Input: part model. Units: mm. Frame: model coordinates. A direction names the side the tool comes from. Coordinates: 2 decimals unless noted, no trailing zeros. Write each loop counter-clockwise with the first axis right and the second up, starting at its lowest first coordinate (ties: lowest second). Pieces come first, ordered by that corner, then holes. Notation, with made-up numbers: M 77.5,38 L 100.5,38 A35 cw 100.5,73 Z; hole C 32,-17 d1. An arc over 180 degrees is marked long. Use CSV: the item, a comma, the result in double quotes.
```python
from build123d import *

# Parameters (mm, degrees)
F0_R     = 5
F0_R_2   = 4.7625
F1_DEPTH = 5
F2_R     = 95
F2_R_2   = 92.5
F3_DEPTH = 38.23
F6_D     = 1.9939
F6_DEPTH = 13.58625
F6_TIP   = 0.5990279941
F7_D     = 10.0838
F7_DEPTH = 13.59
F7_TIP   = 3.0294791551


with BuildPart() as f1:
    # F0 (on Top) → F1 (new body)
    with BuildSketch(Plane.XY):
        with BuildLine():
            ThreePointArc((54.15, -78.0562457463), (84.1702144467, -44.0496878536), (95, 0))
            ThreePointArc((95, 0), (84.1702144467, 44.0496878536), (54.15, 78.0562457463))
            ThreePointArc((54.15, 78.0562457463), (0, 95), (-54.15, 78.0562457463))
            ThreePointArc((-54.15, 78.0562457463), (-95, 0), (-54.15, -78.0562457463))
            ThreePointArc((-54.15, -78.0562457463), (0, -95), (54.15, -78.0562457463))
        make_face()
        Circle(F0_R, mode=Mode.SUBTRACT)
        with BuildLine():
            ThreePointArc((54.15, 78.0562457463), (84.1702144467, 44.0496878536), (95, 0))
            ThreePointArc((95, 0), (84.1702144467, -44.0496878536), (54.15, -78.0562457463))
            Line((54.15, -78.0562457463), (138.5375, -19.5140614366))
            ThreePointArc((138.5375, -19.5140614366), (101.25, 0), (138.5375, 19.5140614366))
            Line((138.5375, 19.5140614366), (54.15, 78.0562457463))
        make_face()
        with BuildLine():
            ThreePointArc((-54.15, -78.0562457463), (-95, 0), (-54.15, 78.0562457463))
            Line((-54.15, 78.0562457463), (-138.5375, 19.5140614366))
            ThreePointArc((-138.5375, 19.5140614366), (-113.9875780366, 21.0425536117), (-101.25, 0))
            ThreePointArc((-101.25, 0), (-113.9875780366, -21.0425536117), (-138.5375, -19.5140614366))
            Line((-138.5375, -19.5140614366), (-54.15, -78.0562457463))
        make_face()
        with BuildLine():
            ThreePointArc((148.75, 0), (146.0425536117, 11.0124219634), (138.5375, 19.5140614366))
            ThreePointArc((138.5375, 19.5140614366), (101.25, 0), (138.5375, -19.5140614366))
            ThreePointArc((138.5375, -19.5140614366), (146.0425536117, -11.0124219634), (148.75, 0))
        make_face()
        with Locations((125, 0)):
            Circle(F0_R_2, mode=Mode.SUBTRACT)
        with BuildLine():
            ThreePointArc((-101.25, 0), (-113.9875780366, 21.0425536117), (-138.5375, 19.5140614366))
            ThreePointArc((-138.5375, 19.5140614366), (-148.75, 0), (-138.5375, -19.5140614366))
            ThreePointArc((-138.5375, -19.5140614366), (-113.9875780366, -21.0425536117), (-101.25, 0))
        make_face()
        with Locations((-125, 0)):
            Circle(F0_R_2, mode=Mode.SUBTRACT)
    extrude(amount=F1_DEPTH)

    # F2 (on face) → F3 (join)
    with BuildSketch(Plane(origin=(0, 0, 0), x_dir=(1, 0, 0), z_dir=(0, 0, -1))):
        Circle(F2_R)
        Circle(F2_R_2, mode=Mode.SUBTRACT)
    extrude(amount=F3_DEPTH)

    # F6
    with Locations(Plane.XY.offset(5)):
        with Locations((-5.75, 5.75), (5.75, 5.75), (5.75, -5.75), (-5.75, -5.75)):
            Hole(F6_D / 2, depth=F6_DEPTH)
            with Locations((0, 0, -(F6_DEPTH + F6_TIP / 2))):  # 118° drill point
                Cone(0, F6_D / 2, F6_TIP, mode=Mode.SUBTRACT)

    # F7
    with Locations(Plane.XY.offset(5)):
        with Locations((-31.75, 0), (31.75, 0)):
            Hole(F7_D / 2, depth=F7_DEPTH)
            with Locations((0, 0, -(F7_DEPTH + F7_TIP / 2))):  # 118° drill point
                Cone(0, F7_D / 2, F7_TIP, mode=Mode.SUBTRACT)


solid = f1.part
```
1. Section C-C (y = -48.5). Return loops of the section in (x, z).
Resolved:
outline,"M -96.75,0 L -81.69,0 L -81.69,-38.23 L -78.77,-38.23 L -78.77,0 L 78.77,0 L 78.77,-38.23 L 81.69,-38.23 L 81.69,0 L 96.75,0 L 96.75,5 L -96.75,5 Z"
2. Section B-B (z = -4.5). Return loops of the section in (x, y).
Resolved:
outline,"C 0,0 d190; hole C 0,0 d185"
3. Material intervals for line 1 (Y direction, x = 0, z = -25); line 2 (Y direction, x = -5.75, z = 2.45); line 3 (Z direction, x = 136.5, y = 2), sorted ascending. Write a range as [from, to].
Resolved:
line 1,"y = [-95, -92.5], [92.5, 95]"
line 2,"y = [-94.83, -6.75], [-4.75, 4.75], [6.75, 94.83]"
line 3,"z = [0, 5]"
4. Section D-D (x = 76.5). Return loops of the section in (y, z), then the cut area to 3 significant figures.
Resolved:
outline,"M -62.55,0 L -56.33,0 L -56.33,-38.23 L -52,-38.23 L -52,0 L 52,0 L 52,-38.23 L 56.33,-38.23 L 56.33,0 L 62.55,0 L 62.55,5 L -62.55,5 Z"
area,"956 mm^2"
5. Section A-A (x = 125). Return loops of the section in (y, z).
Resolved:
outline,"M -28.91,0 L -4.76,0 L -4.76,5 L -28.91,5 Z; M 4.76,0 L 28.91,0 L 28.91,5 L 4.76,5 Z"
6. Access query for faces 1 (the flat face through (-2, 22, 5)), 2 (the flat face through (-1, -19, 0)). Directions: +Z, -Z, +X, -X, +Y, -Y. A direction counts if a zero-diameter tool reaches every point of the face in a straight line with its end or side. Return the directions, or none.
Resolved:
face 1,"+Z, +X, -X, +Y, -Y"
face 2,"-Z"
7. Mould query, pull axis X, two halves, no side actions, for faces 3 (the cylindrical face through (-1.08, -4.88, 2.46)), 4 (the flat face through (-95.753, 49.195, 2.465)), 5 (the flat face through (96.9, 48.4, 2.5)). Classes: pulls with the +X half, pulls with the -X half, needs draft (parallel to the pull), parting line crosses it, or undercut.
Resolved:
face 3,"undercut"
face 4,"pulls with the -X half"
face 5,"pulls with the +X half"
8. Contact query for flat-ended pins moving along their axis: pin 1 Ø10 at (y, z) = (-45, -9.5) entering from +X; pin 2 Ø12 at (x, z) = (66, -33) entering from +Y; pin 3 Ø8 at (x, z) = (52.5, -23.5) entering from -Y. Output: stop coordinate, or through.
Resolved:
pin 1,"stops at x = 86.17"
pin 2,"stops at y = 73.65"
pin 3,"stops at y = -81.69"
